Design review of the part shown in the three views and the two pictorial views. Dimensions are in mm from the part's minimum x, y and z. Coordinates: 2 decimals unless noted, no trailing zeros. Order: outer loops, then holes, each group sorted by start corner. A loop starts at its lowest first (then second) coordinate and runs counter-clockwise, first axis right, second up. Notation, with made-up numbers: (28.5, -2.5) - (67.5, -2.5) arc R19 ccw to (67.5, 24.5) - close; hole circle Ø8 at (82, -21). An arc over 180 degrees is marked (long way). One line per item, written item: value. Start each with the question number.
(1) Consider section A-A on z = 3.5. Write out the cut boundary in (x, y), then the cut area to 3 significant figures.
(2) Consider section D-D on y = 10. Write out the cut boundary in (x, z), then the cut area to 4 significant figures.
(3) Clearance check with flat-ended pins moving along their axes: pin 1 (10 mm diameter, centred on x = 21.5, y = 19.5, fed in from +Z); pin 2 (4 mm diameter, centred on x = 5.5, y = 25, fed in from +Z); pin 3 (6 mm diameter, centred on x = 36.5, y = 16, fed in from +Z); pin 4 (1 mm diameter, centred on y = 19.5, z = 7, fed in from -X). State where each tip first meets the part, or that it passes through.
(4) Mouldability with a two-part tool opening along X and no side actions: class the marked faces 1, 2, 3 and 4 as released by +X, released by -X, zero draft, split by the parting line, or undercut.
(5) Consider section C-C on x = 39.5. Write out the cut boundary in (y, z).
(6) To check wall thickness, follow line 1 along X through (y, z) = (25, 5); line 2 along Y through (x, z) = (39.5, 5.05); line 3 along Y through (x, z) = (5.5, 3.85). State the ranges of each line that lie inside material, in increasing order.
(7) Consider section B-B on z = 6.5. Write out the cut boundary in (x, y).
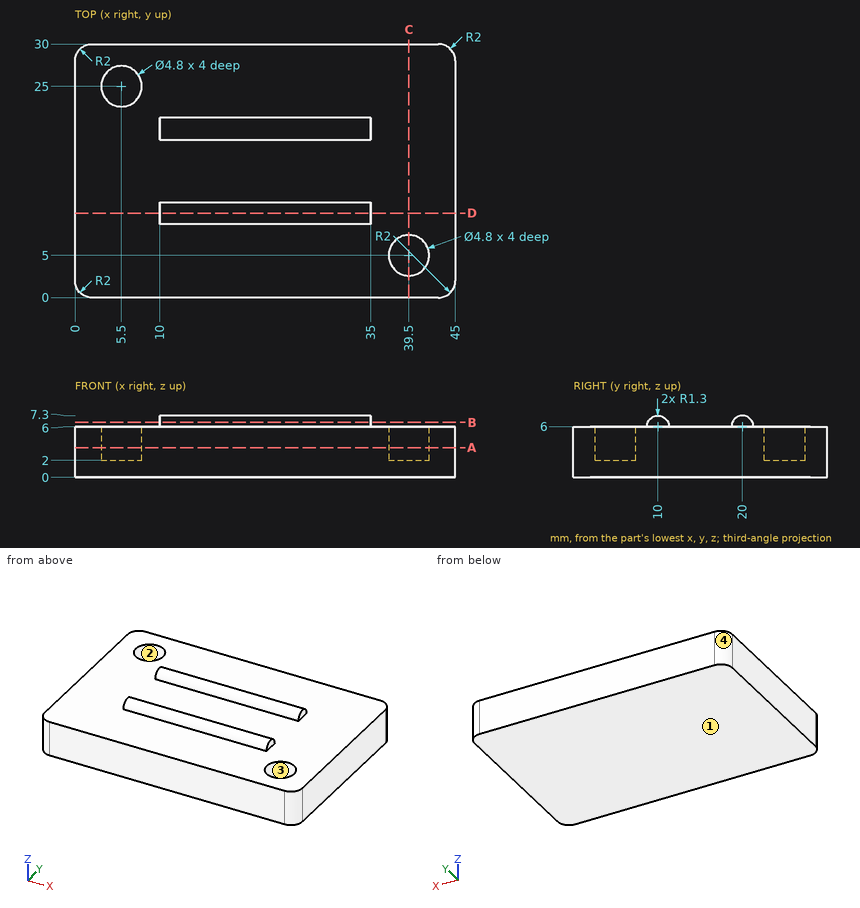
Geometry check:
1. outline: (0, 2) arc R2 ccw to (2, 0) - (43, 0) arc R2 ccw to (45, 2) - (45, 28) arc R2 ccw to (43, 30) - (2, 30) arc R2 ccw to (0, 28) - close; hole circle Ø4.8 at (5.5, 25); hole circle Ø4.8 at (39.5, 5)
1. area: 1,310 mm^2
2. outline: (0, 0) - (45, 0) - (45, 6) - (35, 6) - (35, 7.3) - (10, 7.3) - (10, 6) - (0, 6) - close
2. area: 302.5 mm^2
3. pin 1: stops at z = 7.3
3. pin 2: stops at z = 2
3. pin 3: stops at z = 6
3. pin 4: stops at x = 10
4. face 1: zero draft
4. face 2: undercut
4. face 3: undercut
4. face 4: released by -X
5. outline: (0, 0) - (30, 0) - (30, 6) - (7.4, 6) - (7.4, 2) - (2.6, 2) - (2.6, 6) - (0, 6) - close
6. line 1: x = 0 to 3.1, 7.9 to 45
6. line 2: y = 0 to 2.6, 7.4 to 30
6. line 3: y = 0 to 22.6, 27.4 to 30
7. outline: (10, 8.8) - (35, 8.8) - (35, 11.2) - (10, 11.2) - close; (10, 18.8) - (35, 18.8) - (35, 21.2) - (10, 21.2) - close
